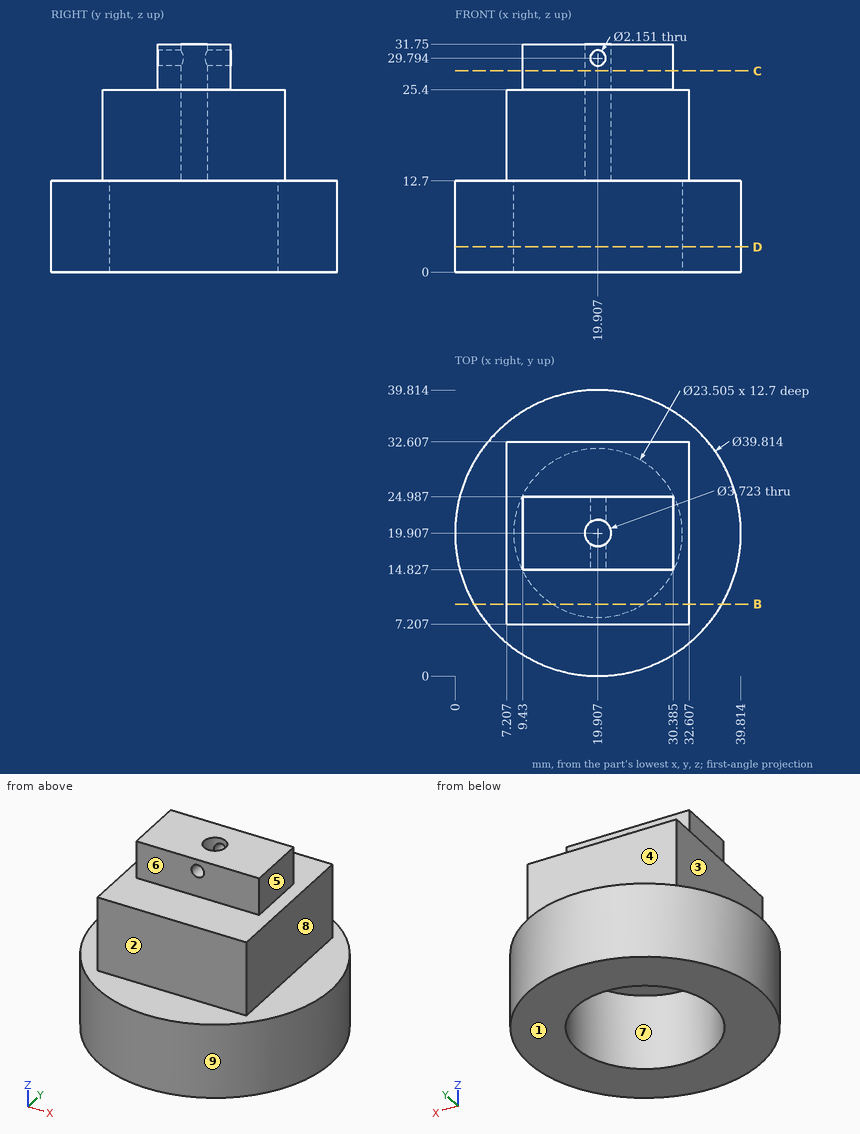
Geometry check sheet. Reference: drawing and pictorial views, mm from the part's lowest x, y, z. A direction names the side the tool comes from. Round coordinates to 2 decimals unless told otherwise and drop trailing zeros. Write each loop counter-clockwise with the first axis right and the second up, starting at its lowest first coordinate (ties: lowest second). Pieces come first, ordered by that corner, then holes. Notation, with made-up numbers: (87, -11.5) -> (120, -11.5) arc R22 ccw to (120, 23.5) -> close; hole circle Ø2 at (-15.5, 27.5). An arc over 180 degrees is marked (long way). Put each result on its own line as item: value.
1) Cross-section at C-C, the plane z = 28. Enter the section's corners in (x, y) (1 decimal), plus the area to 3 significant figures.
Recorded:
outline: (9.4, 14.8) -> (30.4, 14.8) -> (30.4, 25) -> (9.4, 25) -> close; hole circle Ø3.7 at (19.9, 19.9)
area: 202 mm2
2) Release check for a two-part mould opening along Y. For the marked faces 6, 7, 8 and 9 record: pulls with the +Y half, pulls with the -Y half, needs draft (parallel to the pull), parting line crosses it, or undercut.
Recorded:
face 6: pulls with the -Y half
face 7: undercut
face 8: needs draft
face 9: parting line crosses it
3) Cross-section at B-B, the plane y = 10. Enter the section's corners in (x, z) (1 decimal).
Recorded:
outline: (2.6, 0) -> (13.6, 0) -> (13.6, 12.7) -> (26.2, 12.7) -> (26.2, 0) -> (37.2, 0) -> (37.2, 12.7) -> (32.6, 12.7) -> (32.6, 25.4) -> (7.2, 25.4) -> (7.2, 12.7) -> (2.6, 12.7) -> close
4) Depth check by flat-ended pin: P1, Ø14, axis at y = 20, z = 22, coming from the +X side; P2, Ø8, axis at x = 35, z = 6, coming from the -Y side; P3, Ø6.5, axis at x = 22, z = 20, coming from the -Y side; P4, Ø1.9, axis at x = 19.91, z = 29.79, coming from the +Y side. Enter the tip coordinate at first touch or a pass-through.
Recorded:
P1: stops at x = 32.61
P2: stops at y = 3.38
P3: stops at y = 7.21
P4: passes through
5) Cross-section at D-D, the plane z = 3.5. Enter the section's corners in (x, y) (1 decimal).
Recorded:
outline: circle Ø39.8 at (19.9, 19.9); hole circle Ø23.5 at (19.9, 19.9)
6) Thickness scan on probe 1 along X at (y, z) = (21, 17.5) (1 decimal); probe 2 along Y at (x, z) = (21, 29) (1 decimal); probe 3 along Z at (x, y) = (30, 33). Record the ranges inside material, lowest first. Write a range as from..to.
Recorded:
probe 1: x = 7.2..18.4, 21.4..32.6
probe 2: y = 14.8..18.4, 21.4..25
probe 3: z = 0..12.7
7) Access from +Z, -Z, +X, -X, +Y, -Y to the whole of each face (thin tool, end or side, straight path). Record for the marked faces 1, 2, 3, 4 and 5.
Recorded:
face 1: -Z, +X, -X, +Y, -Y
face 2: +Z, +X, -X, -Y
face 3: +Z, -X, +Y, -Y
face 4: +Z, +X, -X, +Y
face 5: +Z, +X, +Y, -Y
